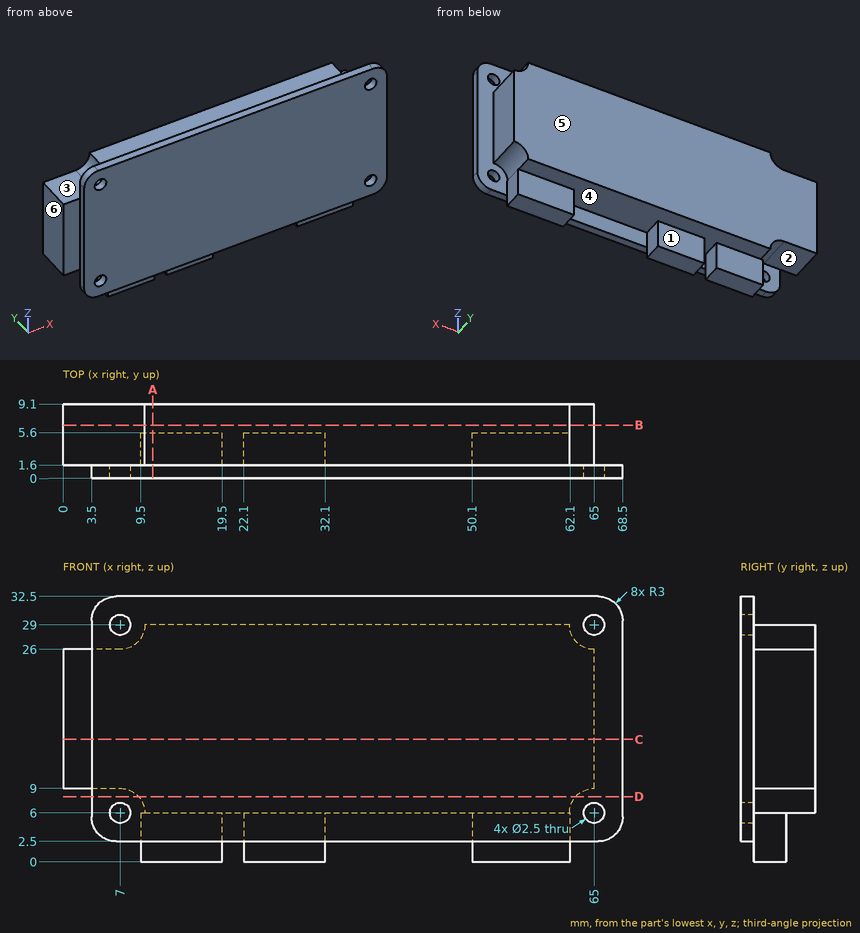
For this review, use the dimensioned drawing (mm, ordinates from the lowest corner) and the shaded views. A direction names the side the tool comes from. Give positions to 0.01 mm unless a question says otherwise; leave off trailing zeros. Loops run counter-clockwise (first coordinate to the right, second up) from the corner with the lowest first, then second, coordinate; pieces in that order, holes last.
Item 1: Draft analysis for pull direction X (two halves, no side actions). For the marked faces 4, 5 and 6, state which applies: +X half, -X half, draft (parallel to the pull), parting line (faces both ways), or undercut.
Item 2: Take a section at B-B, the plane y = 6.5. State the section outline as (x, z) points, and give its area (3 significant figures).
Item 3: Take a section at D-D, the plane z = 8. State the section outline as (x, y) points.
Item 4: Tool access review of the marked faces 1, 2 and 3: name each direction out of +Z, -Z, +X, -X, +Y, -Y from which nothing blocks a thin tool from reaching the whole face with its end or side.
Item 5: For line 1 along Z through (x, y) = (65, 0.6); line 2 along X through (y, z) = (8.5, 12); line 3 along Z through (x, y) = (42, 8.25), list the stretches that pass through material, from the lowest coordinate up.
Item 6: Take a section at A-A, the plane x = 11. State the section outline as (y, z) points.
Item 7: Take a section at C-C, the plane z = 15. State the section outline as (x, y) points.
Item 8: Insertion check: pin 1 (1.2 mm diameter, centred on y = 4.5, z = 4, fed in from +X); pin 2 (3 mm diameter, centred on y = 1.5, z = 13.5, fed in from -X); pin 3 (0.5 mm diameter, centred on y = 0.5, z = 17, fed in from -X); pin 4 (1.8 mm diameter, centred on x = 39.5, z = 5, fed in from +Y). Each pin has a flat end and moves straight along its axis. Give the tip position at first contact, or say it passes through.
Calculated:
1. face 4: undercut
1. face 5: draft
1. face 6: -X half
2. outline: (0, 9) - (7, 9) arc R3 cw to (10, 6) - (62, 6) arc R3 cw to (65, 9) - (65, 26) arc R3 cw to (62, 29) - (10, 29) arc R3 cw to (7, 26) - (0, 26) - close
2. area: 1,420 mm2
3. outline: (3.5, 0) - (68.5, 0) - (68.5, 1.6) - (62.76, 1.6) - (62.76, 9.1) - (9.24, 9.1) - (9.24, 1.6) - (3.5, 1.6) - close
4. face 1: -Z, +X, -X, +Y
4. face 2: -Z, -X, +Y
4. face 3: +Z, -X, +Y
5. line 1: z = 2.5 to 4.75, 7.25 to 27.75, 30.25 to 32.5
5. line 2: x = 0 to 65
5. line 3: z = 6 to 29
6. outline: (0, 2.5) - (1.6, 2.5) - (1.6, 0) - (5.6, 0) - (5.6, 6) - (9.1, 6) - (9.1, 29) - (1.6, 29) - (1.6, 32.5) - (0, 32.5) - close
7. outline: (0, 1.6) - (3.5, 1.6) - (3.5, 0) - (68.5, 0) - (68.5, 1.6) - (65, 1.6) - (65, 9.1) - (0, 9.1) - close
8. pin 1: stops at x = 62.1
8. pin 2: stops at x = 0
8. pin 3: stops at x = 3.5
8. pin 4: stops at y = 1.6
